Source: CAD feature listing. Evaluate the final solid. Frame: model axes, mm. A direction names the side the tool comes from. Coordinates: 2 decimals unless noted, no trailing zeros. Order: outer loops, then holes, each group sorted by start corner. A loop starts at its lowest first (then second) coordinate and runs counter-clockwise, first axis right, second up.
Item 1: Ray query, line 1 (Y direction, x = 0, z = 1.7); line 2 (Y direction, x = 0, z = 12); line 3 (X direction, y = -4.5, z = 1.5). Return the intervals inside material, ascending.
Item 2: Section D-D on z = 9.5. Return the cut outline in (x, y), then the cut area to 3 significant figures.
Item 3: Mould query, pull axis X, two halves, no side actions, for faces 4 (the cylindrical face through (-14.985, 0.66, 2.014)), 5 (the flat face through (0, 8, 17.198)), 6 (the flat face through (3, -8, 5.8)). Classes: released by +X, released by -X, zero draft, split by the parting line, or undercut.
Item 4: Section A-A on x = 0. Return the cut outline in (y, z), then the cut area to 3 significant figures.
Item 5: Section C-C on z = 4.75. Return the cut outline in (x, y).
Item 6: Contact query for flat-ended pins moving along their axis: P1, Ø8, axis at x = 9, y = 3, coming from the -Z side; P2, Ø2, axis at x = -6, y = -11, coming from the -Z side; P3, Ø1, axis at x = 6, y = 8.5, coming from the -Z side; P4, Ø5, axis at y = 3.5, z = 6, coming from the +X side. Output: stop coordinate, or through.
Item 7: Reachability of faces 1 (the flat face through (7.3, -2.4, 0)), 2 (the cylindrical face through (-12.574, 0.553, 10.121)), 3 (the cylindrical face through (-1.86, 14.18, 2.01)) from +Z, -Z, +X, -X, +Y, -Y: full face, straight path, thin tool, end or side. Return the list, or none.
from build123d import *

# Parameters (mm, degrees)
F0_R     = 15
F1_DEPTH = 6.5
F2_R     = 2.4142135624
F4_D     = 15
F5_T     = -0.7
F7_DEPTH = 10.6984395534
F8_R     = 3.3542973282


with BuildPart() as f1:
    # F0 (on Top) → F1 (new body)
    with BuildSketch(Plane.XY):
        Circle(F0_R)
    extrude(amount=F1_DEPTH)

    # F2
    f2_edges = [f1.edges().sort_by_distance(p)[0] for p in [
        (-15, 0, 6.5),
    ]]
    fillet(f2_edges, radius=F2_R)

    # F4 (through all)
    with Locations(Plane(origin=(0, 0, 0), x_dir=(1, 0, 0), z_dir=(0, 0, -1))):
        with Locations((0, 0)):
            Hole(F4_D / 2)

    # F5
    f5_openings = [f1.faces().sort_by_distance(p)[0] for p in [
        (-14.575736, 0, 0),
    ]]
    offset(amount=F5_T, openings=f5_openings)

    # F7 (add): a face of the model
    f7_faces = [f1.faces().sort_by_distance(p)[0] for p in [
        (-12.2298066402, 0, 6.5),
    ]]
    extrude(f7_faces, amount=F7_DEPTH)

    # F8
    f8_edges = [f1.edges().sort_by_distance(p)[0] for p in [
        (-12.585786, 0, 17.19844),
    ]]
    fillet(f8_edges, radius=F8_R)


solid = f1.part
Answer list:
1. line 1: y = -15 to -14.3, -8.2 to -7.5, 7.5 to 8.2, 14.3 to 15
1. line 2: y = -12.59 to -7.5, 7.5 to 12.59
1. line 3: x = -14.31 to -13.57, -6.85 to -6, 6 to 6.85, 13.57 to 14.31
2. outline: circle Ø25.17 at (0, 0); hole circle Ø15 at (0, 0)
2. area: 321 mm2
3. face 4: split by the parting line
3. face 5: zero draft
3. face 6: undercut
4. outline: (-15, 0) - (-14.3, 0) - (-14.3, 4.09) arc R1.71 cw to (-12.59, 5.8) - (-8.2, 5.8) - (-8.2, 0) - (-7.5, 0) - (-7.5, 17.2) - (-9.23, 17.2) arc R3.35 ccw to (-12.59, 13.84) - (-12.59, 6.5) arc R2.41 ccw to (-15, 4.09) - close; (7.5, 0) - (8.2, 0) - (8.2, 5.8) - (12.59, 5.8) arc R1.71 cw to (14.3, 4.09) - (14.3, 0) - (15, 0) - (15, 4.09) arc R2.41 ccw to (12.59, 6.5) - (12.59, 13.84) arc R3.35 ccw to (9.23, 17.2) - (7.5, 17.2) - close
4. area: 129 mm2
5. outline: circle Ø29.81 at (0, 0); circle Ø16.4 at (0, 0); hole circle Ø28.33 at (0, 0); hole circle Ø15 at (0, 0)
6. P1: stops at z = 0
6. P2: stops at z = 5.52
6. P3: stops at z = 5.8
6. P4: stops at x = 14.9
7. face 1: -Z, +X, -X, +Y, -Y
7. face 2: +Z
7. face 3: -Z
